Geometry: final body of the model. Coordinates: model frame, mm. Coordinates: 2 decimals unless noted, no trailing zeros. Loops run counter-clockwise (first coordinate to the right, second up) from the corner with the lowest first, then second, coordinate; pieces in that order, holes last. Notation, with made-up numbers: (-6.5, 4) - (24.5, 4) arc R25 ccw to (24.5, 43) - close; hole circle Ø8 at (-35.5, -24). An arc over 180 degrees is marked (long way). Answer in a Markdown table with one row per item.
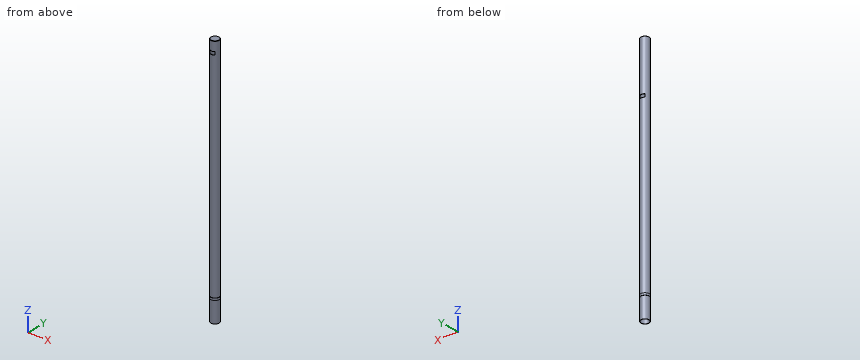
from build123d import *

# Parameters (mm, degrees)
F0_R     = 25.4
F0_R_2   = 23.8125
F1_DEPTH = 1524
F2_DEPTH = 1520.825
F3_SIZE  = 1.5875
F4_W     = 31.75
F4_H     = 19.05
F5_DEPTH = 50.8
F6_START = 127
F0_R_3   = 26.9875
F6_DEPTH = 12.7
F7_DEPTH = 139.7


with BuildPart() as f1:
    # F0 (on Top) → F1 (new body)
    with BuildSketch(Plane.XY):
        Circle(F0_R)
        Circle(F0_R_2, mode=Mode.SUBTRACT)
        Circle(F0_R_2)
    extrude(amount=F1_DEPTH)

    # F0 (on Top) → F2 (cut)
    with BuildSketch(Plane.XY):
        Circle(F0_R_2)
    extrude(amount=F2_DEPTH, mode=Mode.SUBTRACT)

    # F3
    f3_edges = [f1.edges().sort_by_distance(p)[0] for p in [
        (-25.4, 0, 1524),
    ]]
    chamfer(f3_edges, length=F3_SIZE)

    # F4 (on Front) → F5 (cut)
    with BuildSketch(Plane.XZ):
        with Locations((0, 1203.325)):
            Rectangle(F4_W, F4_H)
    extrude(amount=-F5_DEPTH, mode=Mode.SUBTRACT)

    # F0 (on Top) → F6 (join)
    with BuildSketch(Plane.XY.offset(F6_START)):
        Circle(F0_R_3)
        Circle(F0_R, mode=Mode.SUBTRACT)
    extrude(amount=F6_DEPTH)

    # F4 (on Front) → F7 (cut)
    with BuildSketch(Plane.XZ):
        with Locations((0, 1457.325)):
            Rectangle(F4_W, F4_H)
    extrude(amount=F7_DEPTH, mode=Mode.SUBTRACT)


solid = f1.part
(1) Ray query, probe 1 along Y at (x, z) = (1, 1100); probe 2 along Y at (x, z) = (3, 1336); probe 3 along X at (y, z) = (20, 213.5). Return the intervals inside material, ascending.
Verdict:
| item | result |
|---|---|
| probe 1 | y = -25.38 to -23.79, 23.79 to 25.38 |
| probe 2 | y = -25.22 to -23.62, 23.62 to 25.22 |
| probe 3 | x = -15.66 to -12.92, 12.92 to 15.66 |
(2) First-contact query: pin 1 Ø2 at (x, z) = (5.5, 260) entering from +Y; pin 2 Ø0.6 at (y, z) = (18.5, 1206) entering from +X; pin 3 Ø2 at (x, z) = (11, 553.5) entering from +Y. Flat tips, straight axial feed; report the tip coordinate or a pass-through.
Verdict:
| item | result |
|---|---|
| pin 1 | stops at y = 25 |
| pin 2 | stops at x = 17.72 |
| pin 3 | stops at y = 23.35 |
(3) Cut plane C-C on z = 1139. Output: boundary loops of the cut face in (x, y) (1 decimal), then the cut area to 3 significant figures.
Verdict:
| item | result |
|---|---|
| outline | circle Ø50.8 at (0, 0); hole circle Ø47.6 at (0, 0) |
| area | 245 mm² |
(4) Cut plane A-A on x = 0. State how many separate pieces and enclosed holes the cut face has, then the cut area to 3 significant figures.
Verdict:
| item | result |
|---|---|
| separate pieces | 3 |
| enclosed holes | 0 |
| area | 4,970 mm² |
(5) Cut plane B-B on y = 0. Output: boundary loops of the cut face in (x, z) (1 decimal).
Verdict:
| item | result |
|---|---|
| outline | (-27, 127) - (-25.4, 127) - (-25.4, 0) - (-23.8, 0) - (-23.8, 1520.8) - (23.8, 1520.8) - (23.8, 0) - (25.4, 0) - (25.4, 127) - (27, 127) - (27, 139.7) - (25.4, 139.7) - (25.4, 1522.4) - (23.8, 1524) - (-23.8, 1524) - (-25.4, 1522.4) - (-25.4, 139.7) - (-27, 139.7) - close |
